Check sheet for the modelled part. Datum: model origin and axes. Units: mm. A direction names the side the tool comes from. Give positions to 0.01 mm unless a question says otherwise; leave off trailing zeros. Order: outer loops, then holes, each group sorted by start corner. A loop starts at its lowest first (then second) coordinate and runs counter-clockwise, first axis right, second up. Notation, with made-up numbers: (18, 76.5) - (44, 76.5) arc R20 cw to (44, 110.5) - close; hole circle Ø3 at (4.25, 78.5). An arc over 180 degrees is marked (long way). Answer in a Markdown table with one row per item.
Solid Edge part; units mm, degrees
sketch "Sketch1" plane through (0, 0, 0) normal (0, 0, 1) x (1, 0, 0)
  circle A0 centre (0, 0) radius 9.65
  line L0 (-7.0272, -2.0932) -> (-1.7009, -7.1323)
  line L1 (-1.7009, -7.1323) -> (5.3263, -5.0392)
  line L2 (5.3263, -5.0392) -> (7.0272, 2.0932)
  line L3 (7.0272, 2.0932) -> (1.7009, 7.1323)
  line L4 (1.7009, 7.1323) -> (-5.3263, 5.0392)
  line L5 (-5.3263, 5.0392) -> (-7.0272, -2.0932)
extrude "Protrusion1" add sketch "Sketch1" along normal blind 1.5875
properties part number "BumbleB0537"
(1) Gauge pin test, flat end, axial feed: P1, Ø1.5, axis at x = 3, y = -5, coming from the -Z side. Record the tip position at first contact, or that the pin passes through.
Geometry says:
| item | result |
|---|---|
| P1 | z = 0 |
(2) Cross-section at A-A, the plane x = -0.25. Record the cut outline in (y, z), then the cut area to 3 significant figures.
Geometry says:
| item | result |
|---|---|
| outline | (-9.65, 0) - (-6.7, 0) - (-6.7, 1.59) - (-9.65, 1.59) - close; (6.55, 0) - (9.65, 0) - (9.65, 1.59) - (6.55, 1.59) - close |
| area | 9.59 mm² |
(3) Mould release check, pull along X, two halves, no side actions. Record for faces 1 (the flat face through (4.4, 4.58, 0.78)), 2 (the flat face through (6.165, -1.523, 0.783)), 3 (the flat face through (2, -6.3, 1.588)), 4 (the cylindrical face through (9.204, -2.899, 0.783)): pulls with the +X half, pulls with the -X half, needs draft (parallel to the pull), parting line crosses it, or undercut.
Geometry says:
| item | result |
|---|---|
| face 1 | undercut |
| face 2 | undercut |
| face 3 | needs draft |
| face 4 | parting line crosses it |
(4) Thickness scan on L1, parallel to X at y = -4.25, z = 1.05; L2, parallel to X at y = -4.5, z = 1.1; L3, parallel to Y at x = -1.5, z = 0.3. Record the ranges inside material, lowest first.
Geometry says:
| item | result |
|---|---|
| L1 | -8.66 to -4.75, 5.51 to 8.66 |
| L2 | -8.54 to -4.48, 5.45 to 8.54 |
| L3 | -9.53 to -7.07, 6.18 to 9.53 |
(5) Cross-section at B-B, the plane y = 2.75. Record the cut outline in (x, z), then the cut area to 3 significant figures.
Geometry says:
| item | result |
|---|---|
| outline | (-9.25, 0) - (-5.87, 0) - (-5.87, 1.59) - (-9.25, 1.59) - close; (6.33, 0) - (9.25, 0) - (9.25, 1.59) - (6.33, 1.59) - close |
| area | 9.99 mm² |
(6) Cross-section at C-C, the plane z = 0.3. Record the cut outline in (x, y), then the cut area to 3 significant figures.
Geometry says:
| item | result |
|---|---|
| outline | circle Ø19.3 at (0, 0); hole (-7.03, -2.09) - (-1.7, -7.13) - (5.33, -5.04) - (7.03, 2.09) - (1.7, 7.13) - (-5.33, 5.04) - close |
| area | 153 mm² |
(7) Access from +Z, -Z, +X, -X, +Y, -Y to the whole of each face (thin tool, end or side, straight path). Record for faces 5 (the flat face through (1.76, -6.1, 0.78)), 6 (the flat face through (2, -6.3, 0)).
Geometry says:
| item | result |
|---|---|
| face 5 | +Z, -Z |
| face 6 | -Z, +X, -X, +Y, -Y |
(8) Cross-section at D-D, the plane y = -7.75. Record the cut outline in (x, z).
Geometry says:
| item | result |
|---|---|
| outline | (-5.75, 0) - (5.75, 0) - (5.75, 1.59) - (-5.75, 1.59) - close |
